Could you check a few things on this model? Use its own coordinates, in mm. A direction names the side the tool comes from. Coordinates: 2 decimals unless noted, no trailing zeros. Order: outer loops, then holes, each group sorted by start corner. A loop starts at its lowest first (then second) coordinate and runs counter-clockwise, first axis right, second up. Notation, with made-up numbers: (36.25, -2.5) - (67.25, -2.5) arc R29 ccw to (67.25, 20.5) - close; hole circle Ø4 at (72, -10). An arc over 180 degrees is marked (long way). Answer as CSV lines item,"result". Start each with the question number.
1. Thinking about a two-plate mould opening in Z: for faces 1 (the face through (0.206, 0.986, 10.225)), 2 (the face through (1, 1, -14.453)), 3 (the face through (-2.649, 0.986, -8.903)), 4 (the face through (12.317, 1, -4)), which applies, released by +Z, released by -Z, zero draft, split by the parting line, or undercut?
2. I want a section at B-B, the plane y = 0.6. Count the separate pieces of the cut face and the enclosed holes in it, and give its area (3 significant figures).
3. For faces 5 (the face through (1, 1, 5.547)), 6 (the face through (-7, 2, -3)), 7 (the face through (-11, 1, -4.003)), 8 (the face through (11.691, 0.986, -0.316)), 9 (the face through (11, 1, -5.453)), which set-ups out of +Z, -Z, +X, -X, +Y, -Y let a thin tool reach every point of the face, with its end or its side?
4. For pin 1 (3 mm diameter, centred on x = -4, z = 6.5, fed in from -Y); pin 2 (1.2 mm diameter, centred on y = 1, z = 6.5, fed in from -X); pin 3 (0.8 mm diameter, centred on x = 6, y = 1.5, fed in from -Z); pin 4 (1 mm diameter, centred on y = 0.5, z = -2.5, fed in from -X), each with a flat end and sliding along its axis, tell me the tip position at first contact or that it passes through.
5. I want a section at A-A, the plane z = -9.5. List the corners of the cut face in (x, y) for me.
6. I need wall thicknesses on probe 1 along Z at (x, y) = (0, 0.7); probe 2 along Z at (x, y) = (-1.5, 1.35); probe 3 along X at (y, z) = (1.6, -7.75). Which ranges of each line are inside material? Lowest first, please.
from build123d import *

# Parameters (mm, degrees)
BOSS_EXTRUDE1_DEPTH = 2


with BuildPart() as part:
    # Sketch2 → Boss-Extrude1 (new body)
    with BuildSketch(Plane(origin=(0, 0, 0), x_dir=(1, 0, 0), z_dir=(0, 1, 0))):
        with BuildLine():
            Line((-10.683420839, 7.453272885), (-10.683420839, 5.453272885))
            ThreePointArc((-10.683420839, 5.453272885), (-11.183420839, 4.953272885), (-11.683420839, 5.453272885))
            Line((-11.683420839, 5.453272885), (-15.35489401, 5.453272885))
            ThreePointArc((-15.35489401, 5.453272885), (-15.974254556, 5.238379575), (-16.327422226, 4.686057913))
            Line((-16.327422226, 4.686057913), (-18.502568846, -4.401259626))
            ThreePointArc((-18.502568846, -4.401259626), (-18.110467141, -5.448357286), (-16.992741021, -5.477436099))
            Line((-16.992741021, -5.477436099), (-14.606504965, -3.957236073))
            ThreePointArc((-14.606504965, -3.957236073), (-14.453459047, -3.266890545), (-13.76311352, -3.419936464))
            Line((-13.76311352, -3.419936464), (-12.688514303, -5.106719356))
            ThreePointArc((-12.688514303, -5.106719356), (-12.841560222, -5.797064883), (-13.531905749, -5.644018964))
            Line((-13.531905749, -5.644018964), (-16.026002021, -7.232933527))
            ThreePointArc((-16.026002021, -7.232933527), (-16.443355206, -8.374046414), (-15.451333197, -9.075626513))
            Line((-15.451333197, -9.075626513), (-10.493019061, -8.890208712))
            ThreePointArc((-10.493019061, -8.890208712), (-7.77384357, -9.259496243), (-5.339433215, -10.525961738))
            ThreePointArc((-5.339433215, -10.525961738), (-2.723247428, -11.423772675), (-0.091156592, -10.57371951))
            ThreePointArc((-0.091156592, -10.57371951), (0.208841524, -10.219493021), (0.316579161, -9.767975715))
            Line((0.316579161, -9.767975715), (0.316579161, -6.547082806))
            ThreePointArc((0.316579161, -6.547082806), (-0.183420839, -6.047082806), (0.316579161, -5.547082806))
            Line((0.316579161, -5.547082806), (2.316579161, -5.547082806))
            ThreePointArc((2.316579161, -5.547082806), (2.816579161, -6.047082806), (2.316579161, -6.547082806))
            Line((2.316579161, -6.547082806), (2.316579161, -8.930282652))
            ThreePointArc((2.316579161, -8.930282652), (2.563505788, -9.299834465), (2.999421874, -9.213125364))
            Line((2.999421874, -9.213125364), (9.973433411, -2.239113827))
            ThreePointArc((9.973433411, -2.239113827), (11.707615421, 0.356272963), (12.316579161, 3.417740422))
            Line((12.316579161, 3.417740422), (12.316579161, 5.453272885))
            Line((12.316579161, 5.453272885), (10.316579161, 5.453272885))
            ThreePointArc((10.316579161, 5.453272885), (9.816579161, 4.953272885), (9.316579161, 5.453272885))
            Line((9.316579161, 5.453272885), (9.316579161, 7.453272885))
            ThreePointArc((9.316579161, 7.453272885), (9.816579161, 7.953272885), (10.316579161, 7.453272885))
            Line((10.316579161, 7.453272885), (12.316579161, 7.453272885))
            Line((12.316579161, 7.453272885), (12.316579161, 8.202917194))
            ThreePointArc((12.316579161, 8.202917194), (11.437899505, 10.324237538), (9.316579161, 11.202917194))
            Line((9.316579161, 11.202917194), (8.066579161, 11.202917194))
            ThreePointArc((8.066579161, 11.202917194), (6.652365599, 11.788703632), (6.066579161, 13.202917194))
            Line((6.066579161, 13.202917194), (6.066579161, 14.452917194))
            ThreePointArc((6.066579161, 14.452917194), (5.187899505, 16.574237538), (3.066579161, 17.452917194))
            Line((3.066579161, 17.452917194), (2.316579161, 17.452917194))
            Line((2.316579161, 17.452917194), (2.316579161, 15.452917194))
            ThreePointArc((2.316579161, 15.452917194), (2.816579161, 14.952917194), (2.316579161, 14.452917194))
            Line((2.316579161, 14.452917194), (0.316579161, 14.452917194))
            ThreePointArc((0.316579161, 14.452917194), (-0.183420839, 14.952917194), (0.316579161, 15.452917194))
            Line((0.316579161, 15.452917194), (0.316579161, 17.453272885))
            Line((0.316579161, 17.453272885), (-1.718597611, 17.453272885))
            ThreePointArc((-1.718597611, 17.453272885), (-4.78006507, 16.844309145), (-7.37545186, 15.110127135))
            Line((-7.37545186, 15.110127135), (-14.349463397, 8.136115598))
            ThreePointArc((-14.349463397, 8.136115598), (-14.436172498, 7.700199512), (-14.066620685, 7.453272885))
            Line((-14.066620685, 7.453272885), (-11.683420839, 7.453272885))
            ThreePointArc((-11.683420839, 7.453272885), (-11.183420839, 7.953272885), (-10.683420839, 7.453272885))
        make_face()
        with BuildLine():
            Line((-1.133420839, 11.952917194), (-1.133420839, 10.452917194))
            ThreePointArc((-1.133420839, 10.452917194), (-2.683420839, 8.902917194), (-4.233420839, 10.452917194))
            Line((-4.233420839, 10.452917194), (-4.233420839, 11.952917194))
            ThreePointArc((-4.233420839, 11.952917194), (-2.683420839, 13.502917194), (-1.133420839, 11.952917194))
        make_face(mode=Mode.SUBTRACT)
        with BuildLine():
            Line((5.316579161, 4.002917194), (6.816579161, 4.002917194))
            ThreePointArc((6.816579161, 4.002917194), (8.366579161, 2.452917194), (6.816579161, 0.902917194))
            Line((6.816579161, 0.902917194), (5.316579161, 0.902917194))
            ThreePointArc((5.316579161, 0.902917194), (3.766579161, 2.452917194), (5.316579161, 4.002917194))
        make_face(mode=Mode.SUBTRACT)
        with BuildLine():
            Line((-1.133420839, -5.547082806), (-1.133420839, -7.047082806))
            ThreePointArc((-1.133420839, -7.047082806), (-2.683420839, -8.597082806), (-4.233420839, -7.047082806))
            Line((-4.233420839, -7.047082806), (-4.233420839, -5.547082806))
            ThreePointArc((-4.233420839, -5.547082806), (-2.683420839, -3.997082806), (-1.133420839, -5.547082806))
        make_face(mode=Mode.SUBTRACT)
        with BuildLine():
            Line((-10.683420839, 0.902917194), (-12.183420839, 0.902917194))
            ThreePointArc((-12.183420839, 0.902917194), (-13.733420839, 2.452917194), (-12.183420839, 4.002917194))
            Line((-12.183420839, 4.002917194), (-10.683420839, 4.002917194))
            ThreePointArc((-10.683420839, 4.002917194), (-9.133420839, 2.452917194), (-10.683420839, 0.902917194))
        make_face(mode=Mode.SUBTRACT)
        with BuildLine():
            Line((-8.281069122, 0.07251099), (-6.79892731, 1.016739461))
            ThreePointArc((-6.79892731, 1.016739461), (-6.604759329, 1.249227104), (-6.580448639, 1.551155407))
            ThreePointArc((-6.580448639, 1.551155407), (0.690144945, 4.602115628), (-5.147649684, -0.697888449))
            ThreePointArc((-5.147649684, -0.697888449), (-5.431563797, -0.592321001), (-5.724328093, -0.670043431))
            Line((-5.724328093, -0.670043431), (-7.206469905, -1.614271902))
            ThreePointArc((-7.206469905, -1.614271902), (-7.359515824, -2.304617429), (-8.049861351, -2.15157151))
            Line((-8.049861351, -2.15157151), (-9.124460568, -0.464788618))
            ThreePointArc((-9.124460568, -0.464788618), (-8.971414649, 0.225556909), (-8.281069122, 0.07251099))
        make_face(mode=Mode.SUBTRACT)
    extrude(amount=BOSS_EXTRUDE1_DEPTH)


solid = part.part
Solved:
1,face 1,"released by +Z"
1,face 2,"released by -Z"
1,face 3,"undercut"
1,face 4,"zero draft"
2,separate pieces,"1"
2,enclosed holes,"5"
2,area,"487 mm2"
3,face 5,"+Z, +Y, -Y"
3,face 6,"+Z, -Z, +X, -X, +Y"
3,face 7,"+Y, -Y"
3,face 8,"+Z, +X, +Y, -Y"
3,face 9,"+X, +Y, -Y"
4,pin 1,"stops at y = 0"
4,pin 2,"stops at x = -15.82"
4,pin 3,"stops at z = -16.06"
4,pin 4,"stops at x = -16.97"
5,outline,"(-12.99, 0) - (-3.91, 0) - (-3.91, 2) - (-12.99, 2) - close; (-1.46, 0) - (12.02, 0) - (12.02, 2) - (-1.46, 2) - close"
6,probe 1,"z = -17.45 to -15.34, -14.57 to -5.42, 0.51 to 5.66, 6.43 to 10.5"
6,probe 2,"z = -17.45 to -12.95, -9.45 to -6.27, 1.37 to 4.55, 8.05 to 11.26"
6,probe 3,"x = -14.45 to -11.59, -10.78 to 9.41, 10.22 to 12.32"
